Part model, mm, in its own coordinate system. Face numbers are marked on the shaded views. Give positions to 0.01 mm unless a question says otherwise; leave off trailing zeros. Write each loop counter-clockwise with the first axis right and the second up, starting at its lowest first coordinate (ties: lowest second). Pieces come first, ordered by that corner, then holes. Notation, with made-up numbers: M 2,10 L 34,10 A12 ccw 34,30 Z; hole C 11,81 d10. An arc over 180 degrees is marked long. Use CSV: the item, a comma, the result in double quotes. Start each with the question number.
1. Band-saw the part on C-C, the plane z = 1.5. List the corners of the cut face in (x, y).
2. Band-saw the part on D-D, the plane y = 29. List the corners of the cut face in (x, z).
3. Band-saw the part on A-A, the plane y = 0. List the corners of the cut face in (x, z), then the cut area to 3 significant figures.
4. Drill centre lines: line 1 along Y through (x, z) = (-18, 3.65); line 2 along X through (y, z) = (-5.5, 2.65); line 3 along Y through (x, z) = (-20, 5.55). Where is each one in solid material? Low to high. Write a range as from..to.
5. Band-saw the part on B-B, the plane x = -18. List the corners of the cut face in (y, z).
6. Drop flat-ended pins along their axis: pin 1 Ø1.5 at (y, z) = (32, 3.5) entering from +X; pin 2 Ø12.5 at (x, y) = (-18, -31.18) entering from +Z; pin 3 Ø1.5 at (x, z) = (10, 4) entering from +Y. Give the stop position or say it passes through.
7. Mould opens along X. For the marked faces 1, 2, 3 and 4 say: pulls with the +X half, pulls with the -X half, needs draft (parallel to the pull), parting line crosses it, or undercut.
from build123d import *

# Parameters (mm, degrees)
F0_R     = 7
F1_DEPTH = 6
F2_R     = 10


with BuildPart() as f1:
    # F0 (on Top) → F1 (new body)
    with BuildSketch(Plane.XY):
        Polygon((-28.867513, 50), (-28.867513, -50), (57.735027, 0), align=None)
        with Locations((-18, -31.176915)):
            Circle(F0_R, mode=Mode.SUBTRACT)
        Circle(F0_R, mode=Mode.SUBTRACT)
        with Locations((-18, 31.176915)):
            Circle(F0_R, mode=Mode.SUBTRACT)
        with Locations((36, 0)):
            Circle(F0_R, mode=Mode.SUBTRACT)
    extrude(amount=F1_DEPTH)

    # F2
    f2_edges = [f1.edges().sort_by_distance(p)[0] for p in [
        (-28.867513, -50, 3),
        (57.735027, 0, 3),
        (-28.867513, 50, 3),
    ]]
    fillet(f2_edges, radius=F2_R)


solid = f1.part
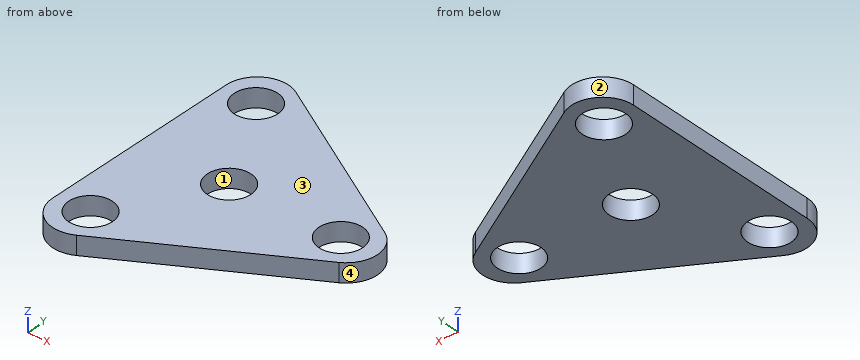
Output:
1,outline,"M -28.87,-32.68 A10 ccw -13.87,-41.34 L 42.74,-8.66 A10 ccw 42.74,8.66 L -13.87,41.34 A10 ccw -28.87,32.68 Z; hole C -18,-31.18 d14; hole C -18,31.18 d14; hole C 0,0 d14; hole C 36,0 d14"
2,outline,"M -28.87,0 L -24.65,0 L -24.65,6 L -28.87,6 Z; M -11.35,0 L 7.51,0 L 7.51,6 L -11.35,6 Z"
3,outline,"M -28.87,0 L -7,0 L -7,6 L -28.87,6 Z; M 7,0 L 29,0 L 29,6 L 7,6 Z; M 43,0 L 47.74,0 L 47.74,6 L 43,6 Z"
3,area,"292 mm²"
4,line 1,"y = -42.64..-38.18, -24.18..24.18, 38.18..42.64"
4,line 2,"x = -28.87..-4.33, 4.33..31.67, 40.33..46.09"
4,line 3,"y = -42.62..-37.89, -24.47..24.47, 37.89..42.62"
5,outline,"M -42.64,0 L -38.18,0 L -38.18,6 L -42.64,6 Z; M -24.18,0 L 24.18,0 L 24.18,6 L -24.18,6 Z; M 38.18,0 L 42.64,0 L 42.64,6 L 38.18,6 Z"
6,pin 1,"stops at x = 3.61"
6,pin 2,"passes through"
6,pin 3,"stops at y = 27.99"
7,face 1,"undercut"
7,face 2,"parting line crosses it"
7,face 3,"needs draft"
7,face 4,"pulls with the +X half"
